Autodesk Inventor part; units mm, degrees
ref_plane "Plano de trabalho2" through (0, 0, 120) normal (0, 0, 1) x (1, 0, 0)
ref_plane "YZ Plane" through (0, 0, 0) normal (1, 0, 0) x (0, 1, 0)
ref_plane "XZ Plane" through (0, 0, 0) normal (0, 1, 0) x (-1, 0, 0)
sketch "Esboço1" plane through (0, 0, 0) normal (0, 0, 1) x (1, 0, 0)
  circle A0 centre (0, 0) radius 55
  dimension "d0" = 110
extrude "Extrusão1" add sketch "Esboço1" along normal blind 20
sketch "Esboço2" plane through (0, 0, 20) normal (0, 0, 1) x (1, 0, 0)
  circle A0 centre (0, 0) radius 44.95
  dimension "d3" = 89.9
ref_plane "Plano de trabalho2" through (0, 0, 120) normal (0, 0, 1) x (1, 0, 0)
sketch "Esboço3" plane through (0, 0, 120) normal (0, 0, 1) x (1, 0, 0)
  circle A0 centre (0, 0) radius 30
  dimension "d6" = 60
loft "Transição1" add profiles "Esboço2", "Esboço3"
fillet "Arredondamento1" radius 34.8 1 edges at (-30, 0, 120)
properties part number "camera"
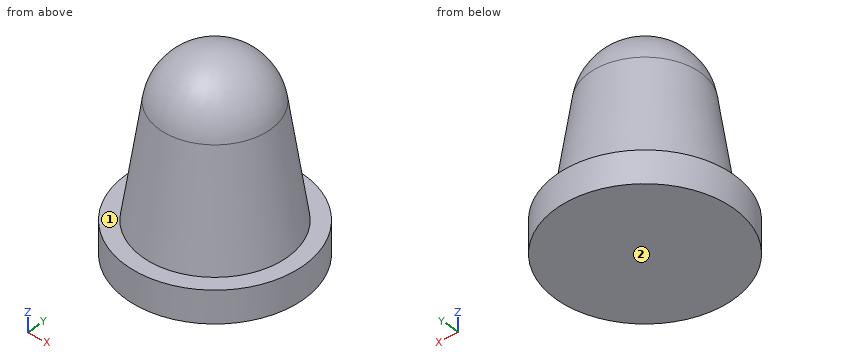
Source: CAD feature listing. Evaluate the final solid. Frame: model axes, mm. Face numbers are marked on the shaded views. A direction names the side the tool comes from. Round coordinates to 2 decimals unless told otherwise and drop trailing zeros. Write item = value, one per line. Start each with the question number.
Item 1: Material intervals for line 1 (Z direction, x = 49, y = -3); line 2 (Z direction, x = -23, y = -22); line 3 (Y direction, x = 29.5, z = 8), sorted ascending.
Item 2: Reachability of the marked faces 1 and 2 from +Z, -Z, +X, -X, +Y, -Y: full face, straight path, thin tool, end or side. Return the list, or none.
Item 3: First-contact query: pin 1 Ø5 at (y, z) = (-24, 44.5) entering from -X; pin 2 Ø1 at (x, z) = (27, 100.5) entering from -Y; pin 3 Ø10 at (y, z) = (16.5, 21.5) entering from +X. Flat tips, straight axial feed; report the tip coordinate or a pass-through.
Results list:
q1.line_1 = 0 to 20
q1.line_2 = 0 to 99.31
q1.line_3 = -46.42 to 46.42
q2.face_1 = +Z
q2.face_2 = -Z, +X, -X, +Y, -Y
q3.pin_1 = -35.31
q3.pin_2 = -16.73
q3.pin_3 = 53.73
